from build123d import *

# Parameters (mm, degrees)
SKETCH1_W           = 47.625
SKETCH1_H           = 152.4
SKETCH1_R           = 14.2875
BOSS_EXTRUDE1_DEPTH = 6.35
CUT_EXTRUDE1_DEPTH  = 81.086188923
SKETCH3_W           = 15.975
SKETCH3_H           = 6.35
BOSS_EXTRUDE2_DEPTH = 6.35
SKETCH4_R           = 1.8288
CUT_EXTRUDE2_DEPTH  = 87.15021855


with BuildPart() as part:
    # Sketch1 → Boss-Extrude1 (new body)
    with BuildSketch(Plane(origin=(0, 0, 0), x_dir=(1, 0, 0), z_dir=(0, 1, 0))):
        Rectangle(SKETCH1_W, SKETCH1_H)
        with Locations(Location((0, 35.5092, 0), (0, 0, 270))):
            Circle(SKETCH1_R, mode=Mode.SUBTRACT)
        with Locations(Location((0, -35.6108, 0), (0, 0, 270))):
            Circle(SKETCH1_R, mode=Mode.SUBTRACT)
    extrude(amount=BOSS_EXTRUDE1_DEPTH)

    # Sketch2 → Cut-Extrude1 (cut, through all)
    with BuildSketch(Plane(origin=(0, 6.35, 0), x_dir=(1, 0, 0), z_dir=(0, 1, 0))):
        with BuildLine():
            ThreePointArc((23.8125, -35.6108), (0, -59.4233), (-23.8125, -35.6108))
            Line((-23.8125, -35.6108), (-23.8125, -76.2))
            Line((-23.8125, -76.2), (23.8125, -76.2))
            Line((23.8125, -76.2), (23.8125, -35.6108))
        make_face()
    extrude(amount=-CUT_EXTRUDE1_DEPTH, mode=Mode.SUBTRACT)

    # Sketch3 → Boss-Extrude2 (add)
    with BuildSketch(Plane(origin=(0, 6.35, 0), x_dir=(1, 0, 0), z_dir=(0, 1, 0))):
        with Locations((-15.825, 79.375)):
            Rectangle(SKETCH3_W, SKETCH3_H)
        with Locations((15.825, 79.375)):
            Rectangle(SKETCH3_W, SKETCH3_H)
    extrude(amount=-BOSS_EXTRUDE2_DEPTH)

    # Sketch4 → Cut-Extrude2 (cut, through all)
    with BuildSketch(Plane(origin=(0, 6.35, 0), x_dir=(1, 0, 0), z_dir=(0, 1, 0))):
        with Locations(Location((-15.875, 79.375, 0), (0, 0, 270))):
            Circle(SKETCH4_R)
        with Locations(Location((15.875, 79.375, 0), (0, 0, 270))):
            Circle(SKETCH4_R)
    extrude(amount=-CUT_EXTRUDE2_DEPTH, mode=Mode.SUBTRACT)


solid = part.part
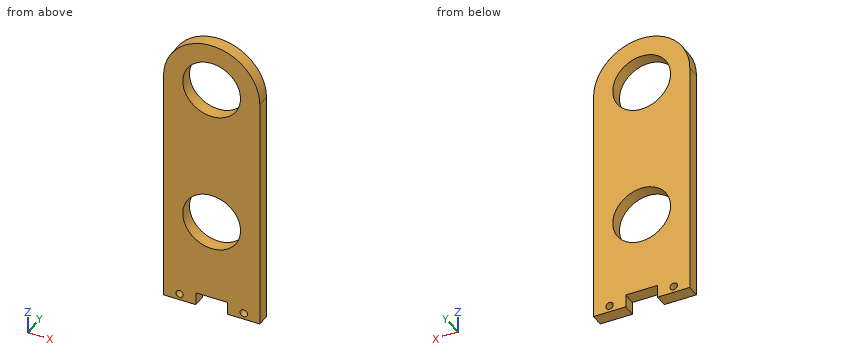
Read the model definition and answer for the solid it produces. Units are mm, in the model's axes. Give positions to 0.01 mm unless a question says otherwise; leave off trailing zeros. Loops run counter-clockwise (first coordinate to the right, second up) from the corner with the lowest first, then second, coordinate; pieces in that order, holes last. Notation, with made-up numbers: (-36, 83.25) -> (-9, 83.25) arc R16 ccw to (-9, 105.25) -> close; hole circle Ø2 at (-5, 25.5). An arc over 180 degrees is marked (long way). Use a Markdown table: item, result.
Q1. Section A-A, the plane x = 0 is taken. Determine the outline of the cut face in (y, z), then the cut area to 3 significant figures.
Solved:
| item | result |
|---|---|
| outline | (0, -76.2) -> (6.35, -76.2) -> (6.35, -49.8) -> (0, -49.8) -> close; (0, -21.22) -> (6.35, -21.22) -> (6.35, 21.32) -> (0, 21.32) -> close; (0, 49.9) -> (6.35, 49.9) -> (6.35, 59.42) -> (0, 59.42) -> close |
| area | 498 mm^2 |
Q2. Section C-C, the plane y = 2 is taken. Count the separate pieces of the cut face and the enclosed holes in it, then the cut area to 3 significant figures.
Solved:
| item | result |
|---|---|
| separate pieces | 1 |
| enclosed holes | 4 |
| area | 5,110 mm^2 |
Q3. Section B-B, the plane z = -36 is taken. Determine the outline of the cut face in (x, y).
Solved:
| item | result |
|---|---|
| outline | (-23.81, 0) -> (-14.28, 0) -> (-14.28, 6.35) -> (-23.81, 6.35) -> close; (14.28, 0) -> (23.81, 0) -> (23.81, 6.35) -> (14.28, 6.35) -> close |
Q4. Find the intervals of material crossed by line 1 along X through (y, z) = (3.5, -35.5); line 2 along Z through (x, y) = (7, 3.5); line 3 along Z through (x, y) = (7.5, 3.25), in increasing order.
Solved:
| item | result |
|---|---|
| line 1 | x = -23.81 to -14.29, 14.29 to 23.81 |
| line 2 | z = -76.2 to -47.96, -23.05 to 23.16, 48.07 to 58.37 |
| line 3 | z = -76.2 to -47.67, -23.35 to 23.45, 47.77 to 58.21 |
